Source: CAD feature listing. Evaluate the final solid. Frame: model axes, mm. Face numbers are marked on the shaded views. A direction names the side the tool comes from. Give positions to 0.01 mm unless a question says otherwise; leave off trailing zeros. Write each loop counter-clockwise with the first axis right and the second up, starting at its lowest first coordinate (ties: lowest second). Pieces come first, ordered by that corner, then holes. Notation, with made-up numbers: (71, 17.5) -> (90, 17.5) arc R9 ccw to (90, 32.5) -> close; hole circle Ø9 at (-21.75, 55). An arc over 180 degrees is marked (long way). Write item = value, one per line.
from build123d import *

# Parameters (mm, degrees)
ESQUISSE1_W        = 10.293411782
ESQUISSE1_H        = 50
BOSS_EXTRU_1_DEPTH = 10
ESQUISSE1_5_W      = 30
ESQUISSE1_5_H      = 10
BOSS_EXTRU_2_DEPTH = 45
ESQUISSE1_6_W      = 10.946693759
ESQUISSE1_6_H      = 50
ESQUISSE1_6_W_2    = 10.293411782
BOSS_EXTRU_3_DEPTH = 10
ESQUISSE1_7_R      = 15
ESQUISSE1_7_R_2    = 12
BOSS_EXTRU_4_DEPTH = 25
ESQUISSE1_8_R      = 15
BOSS_EXTRU_5_DEPTH = 20
CONG_3_R           = 2
CHANFREIN2_SIZE    = 25
CHANFREIN21_SIZE   = 10
CHANFREIN22_SIZE   = 10


with BuildPart() as part:
    # Esquisse1 → Boss.-Extru.1 (new body)
    with BuildSketch(Plane.XY):
        with Locations((-44.853294109, 0)):
            Rectangle(ESQUISSE1_W, ESQUISSE1_H)
    extrude(amount=BOSS_EXTRU_1_DEPTH)

    # Esquisse1<5> → Boss.-Extru.2 (add)
    with BuildSketch(Plane.XY):
        Polygon((-30, 25), (-39.706588218, 25), (-39.706588218, -25), (-30, -25), (-30, -15), (-30, 15), align=None)
        with Locations((-15, -20)):
            Rectangle(ESQUISSE1_5_W, ESQUISSE1_5_H)
        with Locations((-15, 20)):
            Rectangle(ESQUISSE1_5_W, ESQUISSE1_5_H)
    extrude(amount=BOSS_EXTRU_2_DEPTH)

    # Esquisse1<6> → Boss.-Extru.3 (add)
    with BuildSketch(Plane.XY):
        with Locations((44.526653121, 0)):
            Rectangle(ESQUISSE1_6_W, ESQUISSE1_6_H)
        with Locations((-44.853294109, 0)):
            Rectangle(ESQUISSE1_6_W_2, ESQUISSE1_6_H)
    extrude(amount=BOSS_EXTRU_3_DEPTH)


with BuildPart() as boss_extru_3_piece_1:
    # of the separate pieces the step leaves, piece 1, a body of its own (boss_extru_3_pieces)
    add(part.part.solids().sort_by_distance((-50, 25, 0))[0])



with BuildPart() as boss_extru_3_piece_2:
    # of the separate pieces the step leaves, piece 2, a body of its own (boss_extru_3_pieces)
    add(part.part.solids().sort_by_distance((39.053306241, -25, 0))[0])


with BuildPart() as body_3:
    # Esquisse1<7> → Boss.-Extru.4 (new body)
    with BuildSketch(Plane.XY):
        with Locations((15, 0)):
            Circle(ESQUISSE1_7_R)
        with Locations((15, 0)):
            Circle(ESQUISSE1_7_R_2, mode=Mode.SUBTRACT)
    extrude(amount=BOSS_EXTRU_4_DEPTH)


with BuildPart() as boss_extru_3_piece_1_1:
    add(boss_extru_3_piece_1.part)

    add(boss_extru_3_piece_2.part)  # Boss.-Extru.5 merges Boss.-Extru.3 piece 2

    add(body_3.part)  # Boss.-Extru.5 merges body 3
    # Esquisse1<8> → Boss.-Extru.5 (add)
    with BuildSketch(Plane.XY):
        Polygon((39.053306241, 25), (0, 25), (0, 15), (-30, 15), (-30, -15), (0, -15), (0, -25), (39.053306241, -25), align=None)
        with Locations((15, 0)):
            Circle(ESQUISSE1_8_R, mode=Mode.SUBTRACT)
    extrude(amount=BOSS_EXTRU_5_DEPTH)

    # Congé3
    cong_3_edges = [boss_extru_3_piece_1_1.edges().sort_by_distance(p)[0] for p in [
        (0, 0, 20),
    ]]
    fillet(cong_3_edges, radius=CONG_3_R)

    # Chanfrein2
    chanfrein2_edges = [boss_extru_3_piece_1_1.edges().sort_by_distance(p)[0] for p in [
        (0, -20, 45),
    ]]
    chamfer(chanfrein2_edges, length=CHANFREIN2_SIZE - 0.0001)  # a hair under: the kernel refuses the full size

    # Chanfrein21
    chanfrein21_edges = [boss_extru_3_piece_1_1.edges().sort_by_distance(p)[0] for p in [
        (50, 0, 10),
    ]]
    chamfer(chanfrein21_edges, length=CHANFREIN21_SIZE - 0.0001)  # a hair under: the kernel refuses the full size

    # Chanfrein22
    chanfrein22_edges = [boss_extru_3_piece_1_1.edges().sort_by_distance(p)[0] for p in [
        (-50, 0, 10),
    ]]
    chamfer(chanfrein22_edges, length=CHANFREIN22_SIZE - 0.0001)  # a hair under: the kernel refuses the full size


solid = boss_extru_3_piece_1_1.part
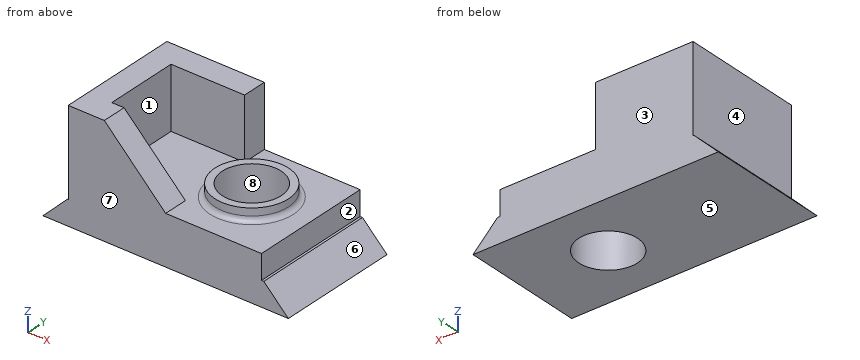
(1) Pull-direction query (X, two-part tool) for the marked faces 6, 7 and 8; classes: pulls with the +X half, pulls with the -X half, needs draft (parallel to the pull), parting line crosses it, or undercut.
Values follow:
face_6 = pulls with the +X half
face_7 = needs draft
face_8 = undercut
(2) First-contact query: pin 1 (1.5 mm diameter, centred on x = 6.5, y = 7.5, fed in from +Z); pin 2 (1 mm diameter, centred on x = 36, y = -0.5, fed in from -Z); pin 3 (5 mm diameter, centred on y = -7, z = 13.5, fed in from +X); pin 4 (11 mm diameter, centred on y = 22, z = 27, fed in from +X). Flat tips, straight axial feed; report the tip coordinate or a pass-through.
Values follow:
pin_1 = 25
pin_2 = 0
pin_3 = 39.05
pin_4 = 0
(3) Material intervals for line 1 (Y direction, x = 15, z = 14); line 2 (X direction, y = -5.5, z = 35.5); line 3 (Z direction, x = 2, y = 19), sorted ascending.
Values follow:
line_1 = -25 to -12, 12 to 25
line_2 = -39.71 to -30
line_3 = 0 to 20
(4) Access query for the marked faces 1, 2, 3, 4 and 5. Directions: +Z, -Z, +X, -X, +Y, -Y. A direction counts if a zero-diameter tool reaches every point of the face in a straight line with its end or side. Return the directions, or none.
Values follow:
face_1 = +Z
face_2 = +Z, +X, +Y, -Y
face_3 = +Z, -Z, +X, -X, +Y
face_4 = +Z, -X, +Y, -Y
face_5 = -Z, +X, -X, +Y, -Y
(5) Section query C-C (z = 15.5). Return loops of the section in (x, y), plus the area to 3 significant figures.
Values follow:
outline = (-39.71, -25) -> (39.05, -25) -> (39.05, 25) -> (-39.71, 25) -> close; hole circle Ø24 at (15, 0)
area = 3,490 mm2
(6) Section query B-B (x = 15). Return loops of the section in (y, z), plus the area to 3 significant figures.
Values follow:
outline = (-25, 0) -> (-12, 0) -> (-12, 25) -> (-15, 25) -> (-15, 22) arc R2 cw to (-17, 20) -> (-25, 20) -> close; (12, 0) -> (25, 0) -> (25, 20) -> (17, 20) arc R2 cw to (15, 22) -> (15, 25) -> (12, 25) -> close
area = 552 mm2
(7) Section query D-D (x = -28). Return loops of the section in (y, z), plus the area to 3 significant figures.
Values follow:
outline = (-25, 0) -> (25, 0) -> (25, 45) -> (15, 45) -> (15, 20) -> (-15, 20) -> (-15, 45) -> (-25, 45) -> close
area = 1,500 mm2
